Autodesk Inventor part; units mm, degrees
ref_plane "YZ Plane" through (0, 0, 0) normal (1, 0, 0) x (0, 1, 0)
ref_plane "XZ Plane" through (0, 0, 0) normal (0, 1, 0) x (-1, 0, 0)
ref_plane "XY Plane" through (0, 0, 0) normal (0, 0, 1) x (1, 0, 0)
sketch "スケッチ1" plane through (0, 0, 0) normal (0, 1, 0) x (-1, 0, 0)
  line L0 (0, 0) -> (70, 0)
  line L1 (70, 0) -> (70, -170)
  line L2 (70, -170) -> (0, -170)
  line L3 (0, -170) -> (0, 0)
  arc A0 (0, -118.5907) -> (0, -26.5907) centre (0, -72.5907) ccw
  arc A1 (0, -128.5907) -> (0, -16.5907) centre (0, -72.5907) ccw
  line L4 (10, -17.4908) -> (0, -17.4908)
  line L5 (0, -17.4908) -> (0, -2.4908)
  line L6 (0, -2.4908) -> (10, -2.4908)
  line L7 (10, -2.4908) -> (10, -17.4908)
  line L8 (10, -127.6907) -> (0, -127.6907)
  line L9 (0, -127.6907) -> (0, -142.6907)
  line L10 (0, -142.6907) -> (10, -142.6907)
  line L11 (10, -142.6907) -> (10, -127.6907)
  line L12 (54.5871, -60.0907) -> (54.5871, -85.0907)
  point P0 (0, -17.4908)
  dimension "d0" = 70
  dimension "d1" = 170
  dimension "d2" = 46
  dimension "d3" = 56
  dimension "d4" = 10
  dimension "d5" = 10
  dimension "d6" = 15
  dimension "d7" = 15
  dimension "d8" = 25
extrude "押し出し1" add sketch "スケッチ1" along normal blind 81 contours L6 L7 A1 L3 | A1 L4 L3 | L4 A1 L12 L8 L3 A0 | L3 A1 L11 L10 | L3 L8 A1
ref_plane "作業平面1" through (-54.5871, 0, -85.0907) normal (-1, 0, 0) x (0, 0, 1)
sketch "スケッチ2" plane through (-54.5871, 0, -85.0907) normal (-1, 0, 0) x (0, 0, 1)
  line L0 (-33.5, 81) -> (58.5, 81)
  line L1 (25, 0) -> (25, 81)
  circle A0 centre (12.5, 40.5) radius 12.5
  line L2 (0, 0) -> (0, 81)
  line L3 (0, 0) -> (25, 0)
  line L4 (-57.5999, 0) -> (-57.5999, 81)
  line L5 (82.5999, 0) -> (82.5999, 81)
  point P0 (85.0907, 0)
  point P1 (12.5, 0)
  point P2 (-57.5999, 40.5)
  point P3 (82.5999, 40.5)
  dimension "d12" = 25
  dimension "d40" = 70.0999
  dimension "d41" = 70.0999
extrude "押し出し2" add sketch "スケッチ2" along normal blind 5 contours A0
ref_plane "作業平面2" through (-59.5871, 40.5, -72.5907) normal (-1, 0, 0) x (0, 0, 1)
ref_plane "作業平面3" through (-10, 0, -142.6907) normal (-1, 0, 0) x (0, 0, 1)
sketch "スケッチ4" plane through (-10, 0, -142.6907) normal (-1, 0, 0) x (0, 0, 1)
  line L0 (0, 81) -> (15, 81)
  line L1 (0, 0) -> (15, 0)
  line L2 (125.1998, 0) -> (140.1998, 0)
  line L3 (125.1998, 81) -> (140.1998, 81)
  point P0 (142.6907, 0)
  point P1 (7.5, 69)
  point P2 (7.5, 12)
  point P3 (132.6998, 12)
  point P4 (132.6998, 69)
  point P5 (7.5, 81)
  point P6 (7.5, 0)
  point P7 (132.6998, 0)
  point P8 (132.6998, 81)
  dimension "d20" = 0
  dimension "d21" = 12
  dimension "d22" = 0
  dimension "d23" = 12
  dimension "d24" = 0
  dimension "d25" = 12
  dimension "d26" = 0
  dimension "d27" = 12
hole "穴1" at (-10, 69, -135.1907) at (-10, 12, -135.1907) at (-10, 12, -9.9908) at (-10, 69, -9.9908) direction (1, 0, 0) diameter 5 end through all
fillet "フィレット1" radius 1 16 edges at (-10, 40.5, -2.4908) (-5, 81, -2.4908) (-10, 81, -9.9908) (-38.6854, 81, -32.1008) (-38.6854, 81, -113.0807) (-10, 81, -135.1907) (-5, 81, -142.6907) (-10, 0, -9.9908) (-38.6854, 0, -32.1008) (-5, 0, -2.4908) (-38.6854, 0, -113.0807) (-54.5871, 0, -72.5907) (-10, 0, -135.1907) (-5, 0, -142.6907) (-10, 40.5, -142.6907) (-54.5871, 81, -72.5907)
sketch "スケッチ8" plane through (-59.5871, 40.5, -72.5907) normal (-1, 0, 0) x (0, 0, 1)
  circle A0 centre (0, 0) radius 8.5
  point P0 (72.5907, -40.5)
  dimension "d46" = 17
extrude "押し出し4" add sketch "スケッチ8" along normal blind 10
sketch "スケッチ9" plane through (-69.5871, 40.5, -72.5907) normal (-1, 0, 0) x (0, 0, 1)
  circle A0 centre (0, 0) radius 8.5
  line L0 (-70.0999, 39.5) -> (-70.0999, -39.5)
  line L1 (12.3865, 40.5) -> (-12.3865, 40.5)
  line L2 (70.0999, -39.5) -> (70.0999, 39.5)
  point P0 (72.5907, -40.5)
  dimension "d49" = 70.0999
  dimension "d50" = 40.5
  dimension "d51" = 70.0999
properties part number "motor_mount2_3D プリント"
Check sheet for the modelled part. Datum: model origin and axes. Units: mm. A direction names the side the tool comes from. Give positions to 0.01 mm unless a question says otherwise; leave off trailing zeros. Order: outer loops, then holes, each group sorted by start corner. A loop starts at its lowest first (then second) coordinate and runs counter-clockwise, first axis right, second up. Notation, with made-up numbers: (3, -18.5) -> (8, -18.5) arc R22 ccw to (8, 11.5) -> close; hole circle Ø8 at (-18.5, -39.5). An arc over 180 degrees is marked (long way). Return JSON: item names as keys, results as strings.
1. Go/stop test with flat-tipped pins: P1, Ø6.5, axis at y = 69, z = -135.19, coming from the -X side; P2, Ø5, axis at x = -37.5, y = 15, coming from the -Z side; P3, Ø12.5, axis at y = 24.5, z = -72, coming from the -X side. Record where each tip stops, or that it passes through.
From the geometry:
{"P1": "x = -10", "P2": "z = -116.31", "P3": "x = -59.59"}
2. Material ranges on probe 1 along Z at (x, y) = (-4, 12); probe 2 along Z at (x, y) = (-2.5, 12); probe 3 along X at (y, z) = (61, -17), recorded low to high. Write a range as [from, to].
From the geometry:
{"probe 1": "[-142.69, -137.69], [-132.69, -118.42], [-26.76, -12.49], [-7.49, -2.49]", "probe 2": "[-142.69, -137.69], [-132.69, -118.52], [-26.66, -12.49], [-7.49, -2.49]", "probe 3": "[-10, 0]"}
3. Cross-section at D-D, the plane z = -72. Record the cut outline in (x, y).
From the geometry:
{"outline": "(-69.59, 32.02) -> (-59.59, 32.02) -> (-59.59, 28.01) -> (-54.59, 28.01) -> (-54.59, 1) arc R1 ccw to (-53.59, 0) -> (-46, 0) -> (-46, 81) -> (-53.59, 81) arc R1 ccw to (-54.59, 80) -> (-54.59, 52.99) -> (-59.59, 52.99) -> (-59.59, 48.98) -> (-69.59, 48.98) -> close"}
4. Cross-section at B-B, the plane x = -6.5. Record the cut outline in (y, z), plus the area to 3 significant figures.
From the geometry:
{"outline": "(0, -141.69) arc R1 ccw to (1, -142.69) -> (80, -142.69) arc R1 ccw to (81, -141.69) -> (81, -118.13) -> (0, -118.13) -> close; (0, -27.05) -> (81, -27.05) -> (81, -3.49) arc R1 ccw to (80, -2.49) -> (1, -2.49) arc R1 ccw to (0, -3.49) -> close; hole circle Ø5 at (12, -135.19); hole circle Ø5 at (12, -9.99); hole circle Ø5 at (69, -135.19); hole circle Ø5 at (69, -9.99)", "area": "3,900 mm^2"}
5. Mould release check, pull along Y, two halves, no side actions. Record for faces 1 (the cylindrical face through (-64.52, 45.67, -79.34)), 2 (the cylindrical face through (-4.9, 70, -132.9)), 3 (the flat face through (-69.587, 41, -73)), 4 (the flat face through (-47, 0, -67)): +Y half, -Y half, draft (parallel to the pull), parting line (faces both ways), or undercut.
From the geometry:
{"face 1": "parting line", "face 2": "undercut", "face 3": "draft", "face 4": "-Y half"}
6. Set-up check for faces 5 (the flat face through (-10, 40, -135)), 6 (the flat face through (-59.587, 32, -70)), 7 (the flat face through (-10, 40, -10)): record each of +Z, -Z, +X, -X, +Y, -Y from which the full face is reachable in a straight line by a thin tool's end or side.
From the geometry:
{"face 5": "-Z, -X, +Y, -Y", "face 6": "-X", "face 7": "+Z, -X, +Y, -Y"}
7. Cross-section at A-A, the plane y = 12. Record the cut outline in (x, z), plus the area to 3 significant figures.
From the geometry:
{"outline": "(-54.59, -85.09) arc R56 ccw to (-10, -127.69) -> (-10, -132.69) -> (0, -132.69) -> (0, -118.59) arc R46 cw to (0, -26.59) -> (0, -12.49) -> (-10, -12.49) -> (-10, -17.49) arc R56 ccw to (-54.59, -60.09) -> close; (-10, -141.69) arc R1 ccw to (-9, -142.69) -> (0, -142.69) -> (0, -137.69) -> (-10, -137.69) -> close; (-10, -7.49) -> (0, -7.49) -> (0, -2.49) -> (-9, -2.49) arc R1 ccw to (-10, -3.49) -> close", "area": "1,770 mm^2"}
8. Cross-section at C-C, the plane y = 25. Record the cut outline in (x, z), plus the area to 3 significant figures.
From the geometry:
{"outline": "(-54.59, -85.09) arc R56 ccw to (-10, -127.69) -> (-10, -141.69) arc R1 ccw to (-9, -142.69) -> (0, -142.69) -> (0, -118.59) arc R46 cw to (0, -26.59) -> (0, -2.49) -> (-9, -2.49) arc R1 ccw to (-10, -3.49) -> (-10, -17.49) arc R56 ccw to (-54.59, -60.09) -> close", "area": "1,870 mm^2"}
